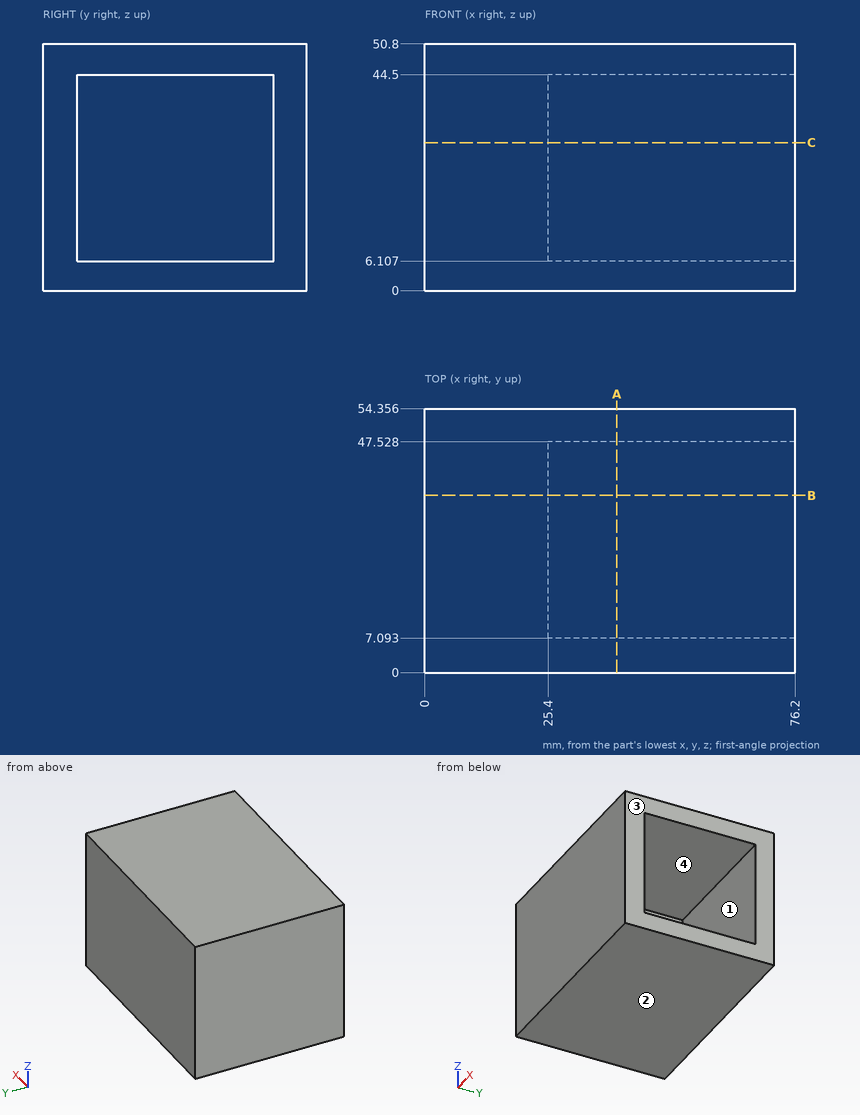
Geometry check sheet. Reference: drawing and pictorial views, mm from the part's lowest x, y, z. Round coordinates to 2 decimals unless told otherwise and drop trailing zeros. Order: outer loops, then holes, each group sorted by start corner. A loop starts at its lowest first (then second) coordinate and runs counter-clockwise, first axis right, second up.
Q1. Cross-section at B-B, the plane y = 36.5. Enter the section's corners in (x, z).
Filled sheet:
outline: (0, 0) - (76.2, 0) - (76.2, 6.11) - (25.4, 6.11) - (25.4, 44.5) - (76.2, 44.5) - (76.2, 50.8) - (0, 50.8) - close
Q2. Cross-section at A-A, the plane x = 39.5. Enter the section's corners in (y, z), plus the area to 3 significant figures.
Filled sheet:
outline: (0, 0) - (54.36, 0) - (54.36, 50.8) - (0, 50.8) - close; hole (7.09, 6.11) - (47.53, 6.11) - (47.53, 44.5) - (7.09, 44.5) - close
area: 1,210 mm2
Q3. Draft check along Z on the marked faces 1, 2, 3 and 4. Enter one of: pulls with the +Z half, pulls with the -Z half, needs draft (parallel to the pull), parting line crosses it, or undercut.
Filled sheet:
face 1: undercut
face 2: pulls with the -Z half
face 3: needs draft
face 4: undercut
Q4. Scan lines: L1, parallel to Z at x = 48, y = 26; L2, parallel to Y at x = 60, z = 31.5; L3, parallel to X at y = 33, z = 25. Record each from-to range of solid material in increasing order.
Filled sheet:
L1: z = 0 to 6.11, 44.5 to 50.8
L2: y = 0 to 7.09, 47.53 to 54.36
L3: x = 0 to 25.4
Q5. Cross-section at C-C, the plane z = 30.5. Enter the section's corners in (x, y), plus the area to 3 significant figures.
Filled sheet:
outline: (0, 0) - (76.2, 0) - (76.2, 7.09) - (25.4, 7.09) - (25.4, 47.53) - (76.2, 47.53) - (76.2, 54.36) - (0, 54.36) - close
area: 2,090 mm2
Q6. Depth check by flat-ended pin: P1, Ø12, axis at y = 32.5, z = 24, coming from the +X side. Enter the tip coordinate at first touch or a pass-through.
Filled sheet:
P1: stops at x = 25.4
